from build123d import *

# Parameters (mm, degrees)
SKETCH1_R           = 2.25
SKETCH1_R_2         = 3.55
BOSS_EXTRUDE1_DEPTH = 4.6


with BuildPart() as part:
    # Sketch1 → Boss-Extrude1 (new body)
    with BuildSketch(Plane(origin=(0, 0, 0), x_dir=(0, 0, -1), z_dir=(1, 0, 0))):
        with BuildLine():
            Line((-21, -10), (6, -10))
            ThreePointArc((6, -10), (8.828427125, -8.828427125), (10, -6))
            Line((10, -6), (10, 19))
            ThreePointArc((10, 19), (8.828427125, 21.828427125), (6, 23))
            Line((6, 23), (-9.695652174, 23))
            ThreePointArc((-9.695652174, 23), (-11.354136506, 22.63997661), (-12.714074263, 21.62471486))
            Line((-12.714074263, 21.62471486), (-24.018422089, 8.62471486))
            ThreePointArc((-24.018422089, 8.62471486), (-24.746577662, 7.401126626), (-25, 6))
            Line((-25, 6), (-25, -6))
            ThreePointArc((-25, -6), (-23.828427125, -8.828427125), (-21, -10))
        make_face()
        with Locations((-15, 0)):
            Circle(SKETCH1_R, mode=Mode.SUBTRACT)
        with Locations((0, 17.25)):
            Circle(SKETCH1_R_2, mode=Mode.SUBTRACT)
        Circle(SKETCH1_R, mode=Mode.SUBTRACT)
    extrude(amount=BOSS_EXTRUDE1_DEPTH)


solid = part.part
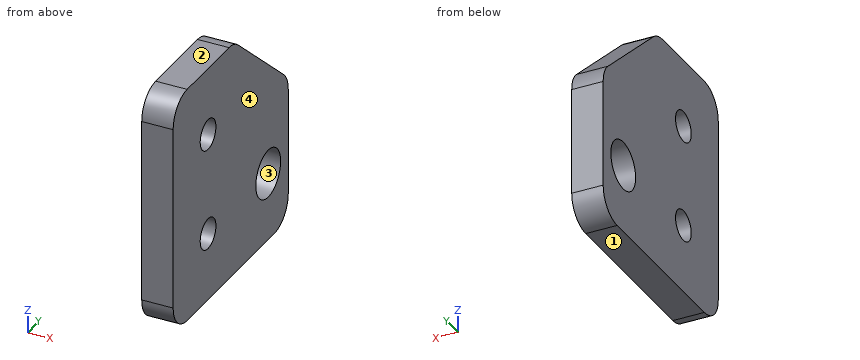
The model under review builds one solid part; all positions refer to its coordinate system, in mm. Face numbers are marked on the shaded views. Round coordinates to 2 decimals unless told otherwise and drop trailing zeros. Order: outer loops, then holes, each group sorted by start corner. A loop starts at its lowest first (then second) coordinate and runs counter-clockwise, first axis right, second up. Notation, with made-up numbers: (62.5, 4) -> (70.5, 4) arc R24 ccw to (70.5, 19) -> close; hole circle Ø5 at (-17.75, -20.5). An arc over 180 degrees is marked (long way). Return JSON: item names as keys, results as strings.
1. Take a section at B-B (y = 0). Write out the cut boundary in (x, z).
Answer block:
{"outline": "(0, -10) -> (4.6, -10) -> (4.6, -2.25) -> (0, -2.25) -> close; (0, 2.25) -> (4.6, 2.25) -> (4.6, 12.75) -> (0, 12.75) -> close; (0, 17.25) -> (4.6, 17.25) -> (4.6, 25) -> (0, 25) -> close"}
2. Insertion check: P1, Ø6, axis at y = -3, z = 15.5, coming from the -X side; P2, Ø3.5, axis at y = 0, z = 15, coming from the +X side. Each pin has a flat end and moves straight along its axis. Give the tip position at first contact, or say it passes through.
Answer block:
{"P1": "stops at x = 0", "P2": "passes through"}
3. The part is to be moulded in two halves that separate along Z. For the marked faces 1, 2, 3 and 4, say which applies: +Z half, -Z half, draft (parallel to the pull), parting line (faces both ways), or undercut.
Answer block:
{"face 1": "-Z half", "face 2": "+Z half", "face 3": "undercut", "face 4": "draft"}
4. Take a section at A-A (z = 0). Write out the cut boundary in (x, y).
Answer block:
{"outline": "(0, -10) -> (4.6, -10) -> (4.6, -2.25) -> (0, -2.25) -> close; (0, 2.25) -> (4.6, 2.25) -> (4.6, 13.7) -> (0, 13.7) -> close; (0, 20.8) -> (4.6, 20.8) -> (4.6, 23) -> (0, 23) -> close"}
5. Take a section at C-C (x = 1.05). Write out the cut boundary in (y, z).
Answer block:
{"outline": "(-10, -6) arc R4 ccw to (-6, -10) -> (19, -10) arc R4 ccw to (23, -6) -> (23, 9.7) arc R4 ccw to (21.62, 12.71) -> (8.62, 24.02) arc R4 ccw to (6, 25) -> (-6, 25) arc R4 ccw to (-10, 21) -> close; hole circle Ø4.5 at (0, 0); hole circle Ø4.5 at (0, 15); hole circle Ø7.1 at (17.25, 0)"}
6. For L1, parallel to Y at x = 1.8, z = 0; L2, parallel to Y at x = 1.5, z = 15; L3, parallel to Y at x = 2.85, z = 2, list the stretches that pass through material, from the lowest coordinate up. Write a range as [from, to].
Answer block:
{"L1": "y = [-10, -2.25], [2.25, 13.7], [20.8, 23]", "L2": "y = [-10, -2.25], [2.25, 19]", "L3": "y = [-10, -1.03], [1.03, 14.32], [20.18, 23]"}
7. Take a section at D-D (z = 15). Write out the cut boundary in (x, y), then the cut area to 3 significant figures.
Answer block:
{"outline": "(0, -10) -> (4.6, -10) -> (4.6, -2.25) -> (0, -2.25) -> close; (0, 2.25) -> (4.6, 2.25) -> (4.6, 19) -> (0, 19) -> close", "area": "113 mm²"}
